Job drawing, mm, ordinate dimensions from the low corner. One solid piece. A direction names the side the tool comes from. Round coordinates to 2 decimals unless told otherwise and drop trailing zeros. Loops run counter-clockwise (first coordinate to the right, second up) from the corner with the lowest first, then second, coordinate; pieces in that order, holes last. Notation, with made-up numbers: M 66.25,75 L 108.25,75 A36 ccw 108.25,110 Z; hole C 50,60.5 d1. An arc over 180 degrees is marked long. Use a Markdown table: item, result. Add a question column.
(1) Which spindle directions (+Z, -Z, +X, -X, +Y, -Y) get a long thin tool onto all of the face, cutting with end or side? Do the marked faces 1, 2 and 3. Say none if no direction does.
(2) Flat gauge pins, fed straight in: P1, Ø1, axis at x = 10.5, z = 17, coming from the +Y side; P2, Ø6, axis at x = 13, y = 5.5, coming from the +Z side; P3, Ø4, axis at y = 9, z = 4, coming from the -X side. Where does each tip first touch, or does it go through?
(3) Band-saw the part on C-C, the plane y = 9.25. Write the cut outline in (x, z), and give its area (3 significant figures).
(4) Band-saw the part on B-B, the plane x = 5. Write the cut outline in (y, z), and give its area (3 significant figures).
(5) Band-saw the part on A-A, the plane z = 1.75. Write the cut outline in (x, y).
(6) Wall check: L1, parallel to Y at x = 5.5, z = 11.75; L2, parallel to Z at x = 12.75, y = 7.25. Give the ranges that are in metal, low to high.
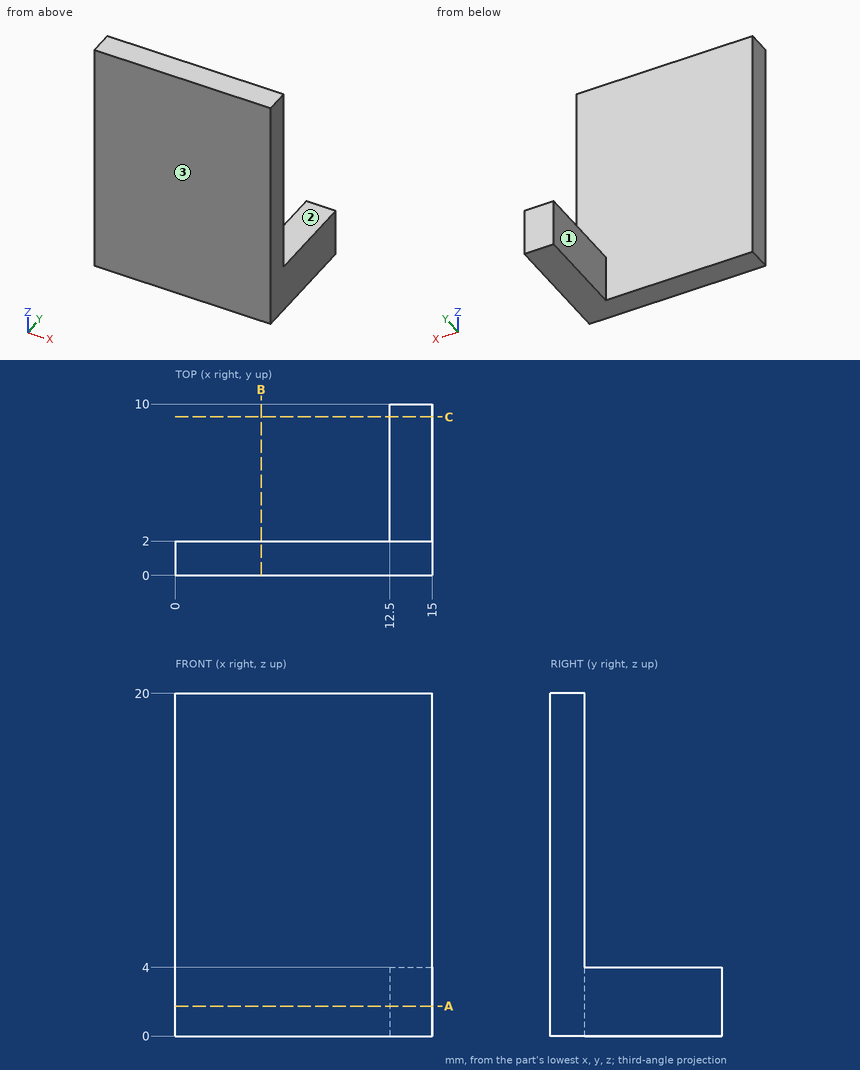
Return value:
| question | item | result |
|---|---|---|
| 1 | face 1 | +Z, -Z, -X, +Y |
| 1 | face 2 | +Z, +X, -X, +Y |
| 1 | face 3 | +Z, -Z, +X, -X, -Y |
| 2 | P1 | y = 2 |
| 2 | P2 | z = 4 |
| 2 | P3 | x = 12.5 |
| 3 | outline | M 12.5,0 L 15,0 L 15,4 L 12.5,4 Z |
| 3 | area | 10.0 mm^2 |
| 4 | outline | M 0,0 L 2,0 L 2,20 L 0,20 Z |
| 4 | area | 40.0 mm^2 |
| 5 | outline | M 0,0 L 15,0 L 15,10 L 12.5,10 L 12.5,2 L 0,2 Z |
| 6 | L1 | 0 to 2 |
| 6 | L2 | 0 to 4 |
